Verification items for the finished model (mm, model axes). A direction names the side the tool comes from. Round coordinates to 2 decimals unless told otherwise and drop trailing zeros. Write each loop counter-clockwise with the first axis right and the second up, starting at its lowest first coordinate (ties: lowest second). Pieces come first, ordered by that corner, then holes. Notation, with made-up numbers: (62, 80.5) - (111, 80.5) arc R34 ccw to (111, 119.5) - close; hole circle Ø2 at (7.25, -26.75). An arc over 180 degrees is marked (long way). Answer as a JSON object with one key per item and string values.
```python
from build123d import *

# Parameters (mm, degrees)
F0_R     = 42.869903
F1_DEPTH = 127
F2_R     = 2.54
F3_R     = 10.834308
F4_DEPTH = 5.08
F5_R     = 1.27


with BuildPart() as f1:
    # F0 (on Front) → F1 (new body)
    with BuildSketch(Plane.XZ):
        Circle(F0_R)
    extrude(amount=F1_DEPTH)

    # F2
    f2_edges = [f1.edges().sort_by_distance(p)[0] for p in [
        (42.869903, -63.5, 0),
        (-42.869903, 0, 0),
        (-42.869903, -127, 0),
    ]]
    fillet(f2_edges, radius=F2_R)

    # F3 (on face) → F4 (join)
    with BuildSketch(Plane.XZ.offset(127)):
        Circle(F3_R)
    extrude(amount=F4_DEPTH)

    # F5
    f5_edges = [f1.edges().sort_by_distance(p)[0] for p in [
        (-10.834308, -132.08, 0),
    ]]
    fillet(f5_edges, radius=F5_R)


solid = f1.part
```
Q1. Set-up check for faces 1 (the flat face through (8, -127, -8)), 2 (the flat face through (-1, 0, 1)): record each of +Z, -Z, +X, -X, +Y, -Y from which the full face is reachable in a straight line by a thin tool's end or side.
Geometry check:
{"face 1": "-Y", "face 2": "+Z, -Z, +X, -X, +Y"}
Q2. Material ranges on line 1 along Y through (x, z) = (-37, 3.5); line 2 along X through (y, z) = (-114, 25.5); line 3 along X through (y, z) = (-76, 26), recorded low to high. Write a range as [from, to].
Geometry check:
{"line 1": "y = [-127, 0]", "line 2": "x = [-34.46, 34.46]", "line 3": "x = [-34.09, 34.09]"}
Q3. Gauge pin test, flat ends, axial feed: P1, Ø1, axis at x = 1, y = -94, coming from the -Z side; P2, Ø6, axis at x = -3, z = -13, coming from the -Y side; P3, Ø1.5, axis at y = -98.5, z = -15, coming from the -X side; P4, Ø1, axis at x = -28, z = -28.5, coming from the +Y side. Record the tip position at first contact, or that the pin passes through.
Geometry check:
{"P1": "stops at z = -42.87", "P2": "stops at y = -131.81", "P3": "stops at x = -40.43", "P4": "stops at y = 0"}
Q4. Section check B-B, the plane x = 0. Record the cut outline in (y, z), then the cut area to 3 significant figures.
Geometry check:
{"outline": "(-132.08, -9.56) arc R1.27 ccw to (-130.81, -10.83) - (-127, -10.83) - (-127, -40.33) arc R2.54 ccw to (-124.46, -42.87) - (-2.54, -42.87) arc R2.54 ccw to (0, -40.33) - (0, 40.33) arc R2.54 ccw to (-2.54, 42.87) - (-124.46, 42.87) arc R2.54 ccw to (-127, 40.33) - (-127, 10.83) - (-130.81, 10.83) arc R1.27 ccw to (-132.08, 9.56) - close", "area": "11,000 mm2"}
Q5. Section check C-C, the plane y = -20.5. Record the cut outline in (x, z).
Geometry check:
{"outline": "circle Ø85.74 at (0, 0)"}
Q6. Section check A-A, the plane z = 0. Record the cut outline in (x, y).
Geometry check:
{"outline": "(-42.87, -124.46) arc R2.54 ccw to (-40.33, -127) - (-10.83, -127) - (-10.83, -130.81) arc R1.27 ccw to (-9.56, -132.08) - (9.56, -132.08) arc R1.27 ccw to (10.83, -130.81) - (10.83, -127) - (40.33, -127) arc R2.54 ccw to (42.87, -124.46) - (42.87, -2.54) arc R2.54 ccw to (40.33, 0) - (-40.33, 0) arc R2.54 ccw to (-42.87, -2.54) - close"}
